Part model, mm, in its own coordinate system. Coordinates: 2 decimals unless noted, no trailing zeros. Write each loop counter-clockwise with the first axis right and the second up, starting at its lowest first coordinate (ties: lowest second). Pieces come first, ordered by that corner, then holes. Notation, with made-up numbers: M -26,86 L 25,86 A34 cw 25,120 Z; hole C 43,30.25 d11. An arc over 180 degrees is marked long. Use a Markdown table: item, result. Add a question column.
Q1. Slice it at C-C on y = 2.5. Write the cut outline in (x, z), then the cut area to 3 significant figures.
Q2. Pin check, flat tip, straight feed: pin 1 Ø3 at (x, y) = (34, 5.5) entering from +Z. Stop position of the tip, or through.
Q3. Mould opens along Y. For faces 1 (the flat face through (26, 0, -10)), 2 (the flat face through (26, 5, -20)), 3 (the cylindrical face through (0.033, 8.33, 0.493)) say: released by +Y, released by -Y, zero draft, split by the parting line, or undercut.
Q4. Slice it at D-D on x = 37. Write the cut outline in (y, z).
Q5. Wall check: L1, parallel to Z at x = 32, y = 5.5. Give the ranges that are in metal, low to high. Write a range as from..to.
from build123d import *

# Parameters (mm, degrees)
SKETCH1_W           = 52
SKETCH1_H           = 20
BOSS_EXTRUDE1_DEPTH = 10
SKETCH3_R           = 0.5
BOSS_EXTRUDE7_DEPTH = 1


with BuildPart() as part:
    # Sketch1 → Boss-Extrude1 (new body)
    with BuildSketch(Plane(origin=(0, 0, 0), x_dir=(1, 0, 0), z_dir=(0, 1, 0))):
        with Locations((26, 10)):
            Rectangle(SKETCH1_W, SKETCH1_H)
    extrude(amount=BOSS_EXTRUDE1_DEPTH)

    # Sketch3 → Boss-Extrude7 (add)
    with BuildSketch(Plane.XY):
        with Locations(Location((0.51, 9.49, 0), (0, 0, 180))):
            Circle(SKETCH3_R)
        with Locations(Location((0.51, 8.48, 0), (0, 0, 180))):
            Circle(SKETCH3_R)
    extrude(amount=BOSS_EXTRUDE7_DEPTH)


solid = part.part
Recorded:
| question | item | result |
|---|---|---|
| 1 | outline | M 0,-20 L 52,-20 L 52,0 L 0,0 Z |
| 1 | area | 1,040 mm² |
| 2 | pin 1 | z = 0 |
| 3 | face 1 | released by -Y |
| 3 | face 2 | zero draft |
| 3 | face 3 | undercut |
| 4 | outline | M 0,-20 L 10,-20 L 10,0 L 0,0 Z |
| 5 | L1 | -20..0 |
